Could you check a few things on this model? Use its own coordinates, in mm. Round coordinates to 2 decimals unless told otherwise and drop trailing zeros. Order: outer loops, then holes, each group sorted by start corner. A loop starts at its lowest first (then second) coordinate and runs counter-clockwise, first axis right, second up. Notation, with made-up numbers: (-31.75, 39.5) - (27.25, 39.5) arc R25 cw to (27.25, 61.5) - close; hole circle Ø6 at (76, 82.5). An arc over 180 degrees is marked (long way). Use one line per item in the form item = value.
from build123d import *

# Parameters (mm, degrees)
SKETCH1_W           = 504
SKETCH1_H           = 425
SKETCH1_R           = 15.08125
BOSS_EXTRUDE1_DEPTH = 19
SKETCH2_R           = 4.25
CUT_EXTRUDE3_DEPTH  = 19


with BuildPart() as part:
    # Sketch1 → Boss-Extrude1 (new body)
    with BuildSketch(Plane(origin=(0, 0, 0), x_dir=(1, 0, 0), z_dir=(0, 1, 0))):
        with Locations((-252, 212.5)):
            Rectangle(SKETCH1_W, SKETCH1_H)
        with Locations(Location((-252, 106.2, 0), (0, 0, 270))):  # turned: the seam where the file's is
            Circle(SKETCH1_R, mode=Mode.SUBTRACT)
    extrude(amount=BOSS_EXTRUDE1_DEPTH)

    # Sketch2 → Cut-Extrude3 (cut)
    with BuildSketch(Plane(origin=(0, 19, 0), x_dir=(1, 0, 0), z_dir=(0, 1, 0))):
        with Locations(Location((-88.599351486, 57.982002922, 0), (0, 0, 270))):  # turned: the seam where the file's is
            Circle(SKETCH2_R)
        with Locations(Location((-14.939385216, 57.911511452, 0), (0, 0, 270))):  # turned: the seam where the file's is
            Circle(SKETCH2_R)
        with Locations(Location((-88.599351486, 13.532002922, 0), (0, 0, 270))):  # turned: the seam where the file's is
            Circle(SKETCH2_R)
        with Locations(Location((-14.939609501, 13.337039706, 0), (0, 0, 270))):  # turned: the seam where the file's is
            Circle(SKETCH2_R)
        with Locations(Location((-14.939609501, 411.662960294, 0), (0, 0, 90))):  # turned: the seam where the file's is
            Circle(SKETCH2_R)
        with Locations(Location((-88.599351486, 411.467997078, 0), (0, 0, 90))):  # turned: the seam where the file's is
            Circle(SKETCH2_R)
        with Locations(Location((-14.939385216, 367.088488548, 0), (0, 0, 90))):  # turned: the seam where the file's is
            Circle(SKETCH2_R)
        with Locations(Location((-88.599351486, 367.017997078, 0), (0, 0, 90))):  # turned: the seam where the file's is
            Circle(SKETCH2_R)
        with Locations(Location((-415.400648514, 367.017997078, 0), (0, 0, 270))):  # turned: the seam where the file's is
            Circle(SKETCH2_R)
        with Locations(Location((-489.060614784, 367.088488548, 0), (0, 0, 270))):  # turned: the seam where the file's is
            Circle(SKETCH2_R)
        with Locations(Location((-415.400648514, 411.467997078, 0), (0, 0, 270))):  # turned: the seam where the file's is
            Circle(SKETCH2_R)
        with Locations(Location((-489.060390499, 411.662960294, 0), (0, 0, 270))):  # turned: the seam where the file's is
            Circle(SKETCH2_R)
        with Locations(Location((-489.060390499, 13.337039706, 0), (0, 0, 90))):  # turned: the seam where the file's is
            Circle(SKETCH2_R)
        with Locations(Location((-415.400648514, 13.532002922, 0), (0, 0, 90))):  # turned: the seam where the file's is
            Circle(SKETCH2_R)
        with Locations(Location((-489.060614784, 57.911511452, 0), (0, 0, 90))):  # turned: the seam where the file's is
            Circle(SKETCH2_R)
        with Locations(Location((-415.400648514, 57.982002922, 0), (0, 0, 90))):  # turned: the seam where the file's is
            Circle(SKETCH2_R)
    extrude(amount=-CUT_EXTRUDE3_DEPTH, mode=Mode.SUBTRACT)


solid = part.part
Item 1: Imagine slicing it at B-B on z = -106.2. Please give me the cut outline in (x, y).
Found:
outline = (-504, 0) - (-267.08, 0) - (-267.08, 19) - (-504, 19) - close; (-236.92, 0) - (0, 0) - (0, 19) - (-236.92, 19) - close
Item 2: If we mould it in two halves opening along X, with no side actions, what happens to faces 1 (the face through (-256, 9, 0)), 2 (the face through (0, 9, -210)), 3 (the face through (-504, 9, -210)), 4 (the face through (-266.723, 9.367, -109.469))? For each: released by +X, released by -X, zero draft, split by the parting line, or undercut.
Found:
face_1 = zero draft
face_2 = released by +X
face_3 = released by -X
face_4 = undercut
Item 3: Imagine slicing it at A-A on x = -252. Please give me the cut outline in (y, z).
Found:
outline = (0, -425) - (19, -425) - (19, -121.28) - (0, -121.28) - close; (0, -91.12) - (19, -91.12) - (19, 0) - (0, 0) - close
Item 4: I need wall thicknesses on L1, parallel to Z at x = -91.5, y = 16.5; L2, parallel to Z at x = -264.5, y = 17.25; L3, parallel to X at y = 10.5, z = -103.5. Which ranges of each line are inside material? Lowest first, please.
Found:
L1 = -425 to -414.57, -408.36 to -370.12, -363.91 to -61.09, -54.88 to -16.64, -10.43 to 0
L2 = -425 to -114.64, -97.76 to 0
L3 = -504 to -266.84, -237.16 to 0
Item 5: Will this pin go through, and if not, where does the flat tip stop? P1, Ø5, axis at x = -415.4, z = -367.02, coming from the -Y side.
Found:
P1 = through
